For this review, take the finished solid that the model builds, in its own axes (mm). A direction names the side the tool comes from. Give positions to 0.01 mm unless a question says otherwise; leave off trailing zeros. Write each loop counter-clockwise with the first axis right and the second up, starting at its lowest first coordinate (ties: lowest second). Pieces come first, ordered by that corner, then holes. Notation, with made-up numbers: (32, 34.25) -> (79, 34.25) arc R11 ccw to (79, 55.25) -> close; hole circle Ø11 at (27.25, 16). An arc over 180 degrees is marked (long way). Return JSON: item names as keys, results as strings.
from build123d import *

# Parameters (mm, degrees)
SKETCH1_W                      = 68
SKETCH1_H                      = 157
BOSS_EXTRUDE1_DEPTH            = 10
M5X0_8_TAPPED_HOLE1_D          = 4.2
M5X0_8_TAPPED_HOLE1_DEPTH      = 12.4
M5X0_8_TAPPED_HOLE1_TIP        = 1.2618073
M4X0_7_TAPPED_HOLE1_AT_2_COUNT = 2
M4X0_7_TAPPED_HOLE1_AT_2_PITCH = 45
CHAMFER1_SIZE                  = 5


with BuildPart() as part:
    # Sketch1 → Boss-Extrude1 (new body)
    with BuildSketch(Plane.XY):
        with Locations((34, 0)):
            Rectangle(SKETCH1_W, SKETCH1_H)
    extrude(amount=-BOSS_EXTRUDE1_DEPTH)

    # M5x0.8 Tapped Hole1
    with Locations(Plane.ZY):
        with Locations((-5, 58.5), (-5, 0), (-5, -58.5)):
            Hole(M5X0_8_TAPPED_HOLE1_D / 2, depth=M5X0_8_TAPPED_HOLE1_DEPTH)
            with Locations((0, 0, -(M5X0_8_TAPPED_HOLE1_DEPTH + M5X0_8_TAPPED_HOLE1_TIP / 2))):  # 118° drill point
                Cone(0, M5X0_8_TAPPED_HOLE1_D / 2, M5X0_8_TAPPED_HOLE1_TIP, mode=Mode.SUBTRACT)

    # Sketch4 → M4x0.7 Tapped Hole1 (revolve, cut)
    with BuildSketch(Plane(origin=(12, 78.5, -5), x_dir=(0, 0, 1), z_dir=(1, 0, 0))):
        Polygon((0, 0), (0, 17.091420021), (1.65, 16.1), (1.65, 0), align=None)
    m4x0_7_tapped_hole1 = revolve(axis=Axis((12, 84.85, -5), (0, -1, 0)), mode=Mode.SUBTRACT)

    # M4x0.7 Tapped Hole1 at 2: M4x0.7 Tapped Hole1 ×2
    with Locations(*[(i * M4X0_7_TAPPED_HOLE1_AT_2_PITCH, 0, 0) for i in range(1, M4X0_7_TAPPED_HOLE1_AT_2_COUNT)]):
        add(m4x0_7_tapped_hole1, mode=Mode.SUBTRACT)

    # Mirror1: M4x0.7 Tapped Hole1 across plane
    add(m4x0_7_tapped_hole1.mirror(Plane.ZX), mode=Mode.SUBTRACT)

    # Mirror1 copy 1 sketch → Mirror1 copy 1 (revolve, cut)
    with BuildSketch(Plane(origin=(57, -78.5, -5), x_dir=(0, 0, 1), z_dir=(1, 0, 0))):
        Polygon((0, 0), (0, -17.091420021), (1.65, -16.1), (1.65, 0), align=None)
    revolve(axis=Axis((57, -84.85, -5), (0, -1, 0)), mode=Mode.SUBTRACT)

    # Chamfer1
    chamfer1_edges = [part.edges().sort_by_distance(p)[0] for p in [
        (0, -78.5, -5),
        (0, 78.5, -5),
    ]]
    chamfer(chamfer1_edges, length=CHAMFER1_SIZE)


solid = part.part
1. To check wall thickness, follow probe 1 along X at (y, z) = (70.75, -5); probe 2 along Y at (x, z) = (5.5, -5); probe 3 along Z at (x, y) = (4.25, 58.5). State the ranges of each line that lie inside material, in increasing order.
Results found:
{"probe 1": "x = 0 to 10.35, 13.65 to 55.35, 58.65 to 68", "probe 2": "y = -78.5 to -60.6, -56.4 to -2.1, 2.1 to 56.4, 60.6 to 78.5", "probe 3": "z = -10 to -7.1, -2.9 to 0"}
2. For pin 1 (2 mm diameter, centred on x = 12, z = -5, fed in from -Y); pin 2 (4 mm diameter, centred on y = 58.5, z = -5, fed in from -X); pin 3 (2.5 mm diameter, centred on x = 57, z = -5, fed in from -Y), all flat-tipped, find the tip position at first contact; note any pin that passes through.
Results found:
{"pin 1": "stops at y = -62.01", "pin 2": "stops at x = 12.46", "pin 3": "stops at y = -62.16"}
3. The part is to be moulded in two halves that separate along X. For faces 1 (the flat face through (2.5, 76, -4.9)), 2 (the flat face through (36, -78.5, -5)), 3 (the cylindrical face through (13, -70.56, -6.31)), 4 (the conical face through (11.76, -61.58, -4.85)), say which applies: +X half, -X half, draft (parallel to the pull), parting line (faces both ways), or undercut.
Results found:
{"face 1": "-X half", "face 2": "draft", "face 3": "undercut", "face 4": "undercut"}
4. Add section A-A, the plane y = 64.5. State the section outline as (x, z) points.
Results found:
{"outline": "(0, -10) -> (68, -10) -> (68, 0) -> (0, 0) -> close; hole circle Ø3.3 at (12, -5); hole circle Ø3.3 at (57, -5)"}
5. For faces 5 (the cylindrical face through (6.29, 56.45, -4.54)), 6 (the flat face through (68, -1, -5)), 7 (the flat face through (34, 1, 0)), 8 (the cylindrical face through (58, 70.56, -6.31)), 9 (the cylindrical face through (58, -70.56, -6.31)), list the 3-axis set-ups (+Z, -Z, +X, -X, +Y, -Y) from which the entire face can be reached by the end or side of a thin tool; tool diameter is ignored.
Results found:
{"face 5": "-X", "face 6": "+Z, -Z, +X, +Y, -Y", "face 7": "+Z, +X, -X, +Y, -Y", "face 8": "+Y", "face 9": "-Y"}
